from build123d import *

# Parameters (mm, degrees)
SKETCH2_W            = 40
SKETCH2_H            = 60
BOSS_EXTRUDE1_DEPTH  = 0.1
SKETCH3_R            = 4
SKETCH3_R_2          = 1.5
BOSS_EXTRUDE2_DEPTH  = 2
BOSS_EXTRUDE5_START  = 5
SKETCH7_R            = 3
SKETCH7_R_2          = 1.5
BOSS_EXTRUDE5_DEPTH  = 5
LPATTERN1_COUNT      = 3
LPATTERN1_PITCH      = 20
LPATTERN1_COUNT_DIR2 = 4
LPATTERN1_PITCH_DIR2 = 20


with BuildPart() as part:
    # Sketch2 → Boss-Extrude1 (new body)
    with BuildSketch(Plane(origin=(0, 0, 0), x_dir=(1, 0, 0), z_dir=(0, 1, 0))):
        with Locations((20, 30)):
            Rectangle(SKETCH2_W, SKETCH2_H)
    extrude(amount=BOSS_EXTRUDE1_DEPTH)

    # Sketch3 → Boss-Extrude2 (add)
    with BuildSketch(Plane(origin=(0, 0.1, 0), x_dir=(1, 0, 0), z_dir=(0, 1, 0))):
        with Locations(Location((0, 0, 0), (0, 0, 90))):
            Circle(SKETCH3_R)
        with Locations(Location((0, 0, 0), (0, 0, 90))):
            Circle(SKETCH3_R_2, mode=Mode.SUBTRACT)
    boss_extrude2 = extrude(amount=BOSS_EXTRUDE2_DEPTH)

    # Sketch7 → Boss-Extrude5 (add)
    with BuildSketch(Plane.XZ.offset(-0.1).offset(BOSS_EXTRUDE5_START)):
        with Locations(Location((0, 0, 0), (0, 0, 270))):
            Circle(SKETCH7_R)
        with Locations(Location((0, 0, 0), (0, 0, 270))):
            Circle(SKETCH7_R_2, mode=Mode.SUBTRACT)
    boss_extrude5 = extrude(amount=-BOSS_EXTRUDE5_DEPTH)

    # LPattern1: Boss-Extrude2, Boss-Extrude5 3 × 4
    with Locations(*[(i * LPATTERN1_PITCH, 0, -j * LPATTERN1_PITCH_DIR2) for i in range(LPATTERN1_COUNT) for j in range(LPATTERN1_COUNT_DIR2) if (i, j) != (0, 0)]):
        add(boss_extrude2)
        add(boss_extrude5)


solid = part.part
Part model, mm, in its own coordinate system. A direction names the side the tool comes from. Coordinates: 2 decimals unless noted, no trailing zeros. Loops run counter-clockwise (first coordinate to the right, second up) from the corner with the lowest first, then second, coordinate; pieces in that order, holes last. Notation, with made-up numbers: M 55.25,64 L 87.25,64 A16 ccw 87.25,89 Z; hole C -8,76.25 d7. An arc over 180 degrees is marked long. Use a Markdown table: item, result. Add a question column.
Q1. Mould opens along Z. For faces 1 (the flat face through (-1.3, -4.9, -1.3)), 2 (the cylindrical face through (36.034, 1.086, 0.521)) say: +Z half, -Z half, draft (parallel to the pull), parting line (faces both ways), or undercut.
Q2. Cut at C-C (x = 12). Write the cut outline in (y, z), and give its area (3 significant figures).
Q3. Which spindle directions (+Z, -Z, +X, -X, +Y, -Y) get a long thin tool onto all of the face, cutting with end or side? Do faces 3 (the flat face through (20, 2.1, -42)), 4 (the cylindrical face through (39.1, -1.4, -18.8)), 5 (the cylindrical face through (42.03, -2.44, -17.79)), 6 (the flat face through (38.7, -4.9, -61.3)), 7 (the cylindrical face through (2.4, 1.1, -16.8)). Say none if no direction does.
Q4. Probe L1, parallel to X at y = -3, z = -60; L2, parallel to X at y = 1.4, z = -40; L3, parallel to X at y = 0.5, z = -43. List the from-to ranges inside material, lowest first.
Q5. Cut at A-A (y = -2). Give the number of separate pieces and of enclosed holes in the cut face, and give its area (3 significant figures).
Q6. Cut at D-D (z = -52). Write the cut outline in (x, y), and give its area (3 significant figures).
Q7. Pin check, flat tips, straight feed: P1, Ø1, axis at x = 36.5, z = -4, coming from the +Y side; P2, Ø1.2, axis at x = 39.5, z = -20.5, coming from the -Y side; P3, Ø3, axis at y = -4, z = -34.5, coming from the +X side. Stop position of each tip, or through.
Worked out:
| question | item | result |
|---|---|---|
| 1 | face 1 | draft |
| 1 | face 2 | undercut |
| 2 | outline | M 0,-60 L 0.1,-60 L 0.1,0 L 0,0 Z |
| 2 | area | 6.00 mm2 |
| 3 | face 3 | +Z, -Z, +X, -X, +Y |
| 3 | face 4 | none |
| 3 | face 5 | -Y |
| 3 | face 6 | +Z, -Z, +X, -X, -Y |
| 3 | face 7 | +Y |
| 4 | L1 | x = -3 to -1.5, 1.5 to 3, 17 to 18.5, 21.5 to 23, 37 to 38.5, 41.5 to 43 |
| 4 | L2 | x = -4 to -1.5, 1.5 to 4, 16 to 18.5, 21.5 to 24, 36 to 38.5, 41.5 to 44 |
| 4 | L3 | x = -2.65 to 2.65, 17.35 to 22.65, 37.35 to 42.65 |
| 5 | separate pieces | 12 |
| 5 | enclosed holes | 12 |
| 5 | area | 254 mm2 |
| 6 | outline | M 0,0 L 40,0 L 40,0.1 L 0,0.1 Z |
| 6 | area | 4.00 mm2 |
| 7 | P1 | stops at y = 0.1 |
| 7 | P2 | stops at y = 0 |
| 7 | P3 | passes through |
